Autodesk Fusion 360 part; units mm, degrees
sketch "Sketch1" plane through (0, 0, 0) normal (0, 1, 0) x (1, 0, 0)
  line L0 (0, 0) -> (6.9459, -39.3923)
  line L1 (0, 0) -> (40, 0) construction
  line L2 (0, 0) -> (5, 0)
  line L3 (6.9459, -39.3923) -> (11.9459, -39.3923)
  line L4 (5, 0) -> (11.9459, -39.3923)
  dimension "d1" = 80
  dimension "d2" = 40
  dimension "d3" = 5
  dimension "d4" = 5
extrude "Extrude1" add sketch "Sketch1" along normal blind 40
sketch "Sketch2" plane through (0, 0, 0) normal (0, 0, -1) x (1, 0, 0)
  line L0 (5, 0) -> (0, 0)
  line L1 (0, 0) -> (0, -40)
  line L2 (0, -40) -> (5, -40)
  line L3 (5, -40) -> (5, 0)
  line L4 (0, -40) -> (0, -38.75)
  line L5 (0, -38.75) -> (0, -38.65)
  line L6 (0, -38.65) -> (1.35, -38.65)
  line L7 (1.35, -38.65) -> (3.65, -38.65)
  line L8 (3.65, -38.65) -> (3.65, -36.35)
  line L9 (3.65, -36.35) -> (1.35, -36.35)
  line L10 (1.35, -36.35) -> (1.35, -38.65)
  line L11 (0, 0) -> (0, -1.35)
  line L12 (0, -1.35) -> (1.35, -1.35)
  line L13 (1.35, -1.35) -> (3.65, -1.35)
  line L14 (3.65, -1.35) -> (3.65, -3.65)
  line L15 (3.65, -3.65) -> (1.35, -3.65)
  line L16 (1.35, -3.65) -> (1.35, -1.35)
  dimension "d7" = 1.25
  dimension "d8" = 0.1
  dimension "d9" = 1.35
  dimension "d10" = 2.3
  dimension "d11" = 2.3
  dimension "d12" = 1.35
  dimension "d13" = 1.35
  dimension "d14" = 2.3
  dimension "d15" = 2.3
extrude "Extrude2" add sketch "Sketch2" along normal blind 5 contours L13 L14 L15 L16 | L7 L8 L9 L10
sketch "Sketch3" plane through (4.8492, 0, -0.8551) normal (0.9848, 0, -0.1736) x (0, 1, 0)
  line L0 (0, 40.8682) -> (0, 0.8682)
  line L1 (0, 0.8682) -> (40, 0.8682)
  line L2 (40, 0.8682) -> (40, 40.8682)
  line L3 (40, 40.8682) -> (0, 40.8682)
  line L4 (5.9613, 40.8682) -> (5.9613, 35.8682)
  line L5 (0, 35.8688) -> (5, 35.8688)
  line L6 (5, 35.8688) -> (5, 35.1188)
  line L7 (5, 35.1188) -> (5.75, 35.1188)
  circle A0 centre (5.75, 35.1188) radius 0.75
  line L8 (5.75, 35.1188) -> (34.25, 35.1188)
  circle A1 centre (34.25, 35.1188) radius 0.75
  line L9 (5.75, 35.1188) -> (5.75, 6.6188)
  circle A2 centre (5.75, 6.6188) radius 0.75
  line L10 (5.75, 6.6188) -> (34.25, 6.6188)
  circle A3 centre (34.25, 6.6188) radius 0.75
  dimension "d18" = 5
  dimension "d19" = 5
  dimension "d20" = 0.75
  dimension "d21" = 0.75
  dimension "d22" = 1.5
  dimension "d23" = 28.5
  dimension "d24" = 1.5
  dimension "d25" = 28.5
  dimension "d26" = 1.5
  dimension "d27" = 28.5
  dimension "d28" = 1.5
extrude "Extrude3" cut sketch "Sketch3" against normal blind 7098 contours A1 | A3 | L9 A2 L10 | L9 A2 L10 | L7 A0 L8 | L7 A0 L9 | A0 L8 L9
Source: CAD feature listing. Evaluate the final solid. Frame: model axes, mm. A direction names the side the tool comes from. Give positions to 0.01 mm unless a question says otherwise; leave off trailing zeros. Loops run counter-clockwise (first coordinate to the right, second up) from the corner with the lowest first, then second, coordinate; pieces in that order, holes last. Notation, with made-up numbers: (-25, -25) -> (3, -25) arc R21 ccw to (3, 4) -> close; hole circle Ø6 at (41.25, 62). An arc over 180 degrees is marked (long way). Use a Markdown table: item, result. Add a question column.
(1) Section query B-B (y = 37). Output: boundary loops of the cut face in (x, z), then the cut area to 3 significant figures.
(2) First-contact query: pin 1 Ø1.5 at (x, y) = (3.5, 14.5) entering from -Z; pin 2 Ø6 at (y, z) = (34.5, 32.5) entering from -X; pin 3 Ø1.5 at (y, z) = (6.5, 34.5) entering from -X; pin 4 Ø5 at (x, z) = (9.5, 30) entering from -Y. Flat tips, straight axial feed; report the tip coordinate or a pass-through.
(3) Ray query, line 1 (X direction, y = 15.5, z = 35); line 2 (X direction, y = 33, z = 16.5). Return the intervals inside material, ascending.
(4) Section query C-C (x = 2). Count the separate pieces of the cut face and the enclosed holes in it, then the cut area to 3 significant figures.
(5) Access query for faces 5 (the face through (3, 36.35, -2)), 6 (the face through (1.35, 37, -2)), 7 (the face through (3.65, 38, -2)), 8 (the face through (2, 38.65, -2)). Directions: +Z, -Z, +X, -X, +Y, -Y. A direction counts if a zero-diameter tool reaches every point of the face in a straight line with its end or side. Return the directions, or none.
(6) Section query D-D (z = 11). Output: boundary loops of the cut face in (x, y), then the cut area to 3 significant figures.
(7) Section query A-A (z = -1). Output: boundary loops of the cut face in (x, y), then the cut area to 3 significant figures.
(8) Pull-direction query (X, two-part tool) for faces 1 (the face through (8.596, 34.965, 34.374)), 2 (the face through (2, 1.35, -2)), 3 (the face through (3.424, 19.72, 19.42)), 4 (the face through (3.65, 2, -2)); classes: +X half, -X half, draft (parallel to the pull), parting line (faces both ways), or undercut.
Checked values:
| question | item | result |
|---|---|---|
| 1 | outline | (0, 0) -> (1.35, 0) -> (1.35, -5) -> (3.65, -5) -> (3.65, 0) -> (5, 0) -> (11.95, 39.39) -> (6.95, 39.39) -> close |
| 1 | area | 208 mm^2 |
| 2 | pin 1 | z = 0 |
| 2 | pin 2 | x = 5.2 |
| 2 | pin 3 | x = 5.95 |
| 2 | pin 4 | y = 0 |
| 3 | line 1 | 6.17 to 11.17 |
| 3 | line 2 | 2.91 to 7.91 |
| 4 | separate pieces | 1 |
| 4 | enclosed holes | 2 |
| 4 | area | 473 mm^2 |
| 5 | face 5 | -Z, +X, -X |
| 5 | face 6 | -Z, -X, +Y, -Y |
| 5 | face 7 | -Z, +X, +Y, -Y |
| 5 | face 8 | -Z, +X, -X, +Y |
| 6 | outline | (1.94, 0) -> (6.94, 0) -> (6.94, 40) -> (1.94, 40) -> close |
| 6 | area | 200 mm^2 |
| 7 | outline | (1.35, 1.35) -> (3.65, 1.35) -> (3.65, 3.65) -> (1.35, 3.65) -> close; (1.35, 36.35) -> (3.65, 36.35) -> (3.65, 38.65) -> (1.35, 38.65) -> close |
| 7 | area | 10.6 mm^2 |
| 8 | face 1 | undercut |
| 8 | face 2 | draft |
| 8 | face 3 | -X half |
| 8 | face 4 | +X half |
